Geometry: final body of the model. Coordinates: model frame, mm. A direction names the side the tool comes from. Round coordinates to 2 decimals unless told otherwise and drop trailing zeros. Loops run counter-clockwise (first coordinate to the right, second up) from the corner with the lowest first, then second, coordinate; pieces in that order, holes last. Notation, with made-up numbers: M 11.5,51.5 L 24.5,51.5 A12 ccw 24.5,71.5 Z; hole C 56,-21 d10. An arc over 180 degrees is marked long. Write each question's results on one line, items separated by ' | '.
```python
from build123d import *

# Parameters (mm, degrees)
SKETCH_1_W          = 40
SKETCH_1_H          = 60
EXTRUDE_1_DEPTH     = 3
SKETCH_2_W          = 40
SKETCH_2_H          = 3
EXTRUDE_2_DEPTH     = 40
EXTRUDE_3_DEPTH     = 23
CUT_EXTRUDE_1_DEPTH = 17


with BuildPart() as part:
    # 草图1 → 凸台-拉伸1 (new body)
    with BuildSketch(Plane.XY):
        with Locations((20, -30)):
            Rectangle(SKETCH_1_W, SKETCH_1_H)
    extrude(amount=EXTRUDE_1_DEPTH)

    # 草图2 → 凸台-拉伸2 (add)
    with BuildSketch(Plane.XY.offset(3)):
        with Locations((20, -41.5)):
            Rectangle(SKETCH_2_W, SKETCH_2_H)
    extrude(amount=EXTRUDE_2_DEPTH)

    # 草图3 → 凸台-拉伸3 (add)
    with BuildSketch(Plane.ZY):
        Polygon((3, -55), (28, -43), (3, -43), align=None)
    extrude(amount=-EXTRUDE_3_DEPTH)

    # 草图3<2> → 切除-拉伸1 (cut)
    with BuildSketch(Plane.ZY):
        Polygon((3, -55), (28, -43), (3, -43), align=None)
    extrude(amount=-CUT_EXTRUDE_1_DEPTH, mode=Mode.SUBTRACT)


solid = part.part
```
1. Section D-D (z = 35.5). Output: boundary loops of the cut face in (x, y), then the cut area to 3 significant figures.
Answer key:
outline: M 0,-43 L 40,-43 L 40,-40 L 0,-40 Z | area: 120 mm²
2. Section C-C (y = -53). Output: boundary loops of the cut face in (x, z), then the cut area to 3 significant figures.
Answer key:
outline: M 0,0 L 40,0 L 40,3 L 23,3 L 23,7.17 L 17,7.17 L 17,3 L 0,3 Z | area: 145 mm²
3. Ray query, probe 1 along Z at (x, y) = (11.5, -32); probe 2 along Y at (x, z) = (9, 6); probe 3 along Y at (x, z) = (19, 22.5). Return the intervals inside material, ascending.
Answer key:
probe 1: z = 0 to 3 | probe 2: y = -43 to -40 | probe 3: y = -45.64 to -40
4. Section A-A (z = 4). Output: boundary loops of the cut face in (x, y), then the cut area to 3 significant figures.
Answer key:
outline: M 0,-43 L 17,-43 L 17,-54.52 L 23,-54.52 L 23,-43 L 40,-43 L 40,-40 L 0,-40 Z | area: 189 mm²
5. Section B-B (x = 20). Output: boundary loops of the cut face in (y, z), then the cut area to 3 significant figures.
Answer key:
outline: M -60,0 L 0,0 L 0,3 L -40,3 L -40,43 L -43,43 L -43,28 L -55,3 L -60,3 Z | area: 450 mm²
6. Access query for faces 1 (the face through (24, -43, 23)), 2 (the face through (17, -48, 13)), 3 (the face through (23, -48, 13)), 4 (the face through (20, -20, 3)). Directions: +Z, -Z, +X, -X, +Y, -Y. A direction counts if a zero-diameter tool reaches every point of the face in a straight line with its end or side. Return the directions, or none.
Answer key:
face 1: +Z, -Y | face 2: +Z, -X, -Y | face 3: +Z, +X, -Y | face 4: +Z, +X, -X, +Y
7. Pin query (flat end, axial travel): P1, Ø12, axis at x = 16, z = 24.5, coming from the +Y side; P2, Ø12, axis at x = 6.5, z = 34.5, coming from the -Y side; P3, Ø13, axis at y = -50, z = 16.5, coming from the -X side. Return the tip coordinate at first contact, or that it passes through.
Answer key:
P1: stops at y = -40 | P2: stops at y = -43 | P3: stops at x = 17
